Autodesk Inventor part; units mm, degrees
ref_plane "YZ Plane" through (0, 0, 0) normal (1, 0, 0) x (0, 1, 0)
ref_plane "XZ Plane" through (0, 0, 0) normal (0, 1, 0) x (-1, 0, 0)
ref_plane "XY Plane" through (0, 0, 0) normal (0, 0, 1) x (1, 0, 0)
sketch "Boceto1" plane through (-15.751, -17.109, 5) normal (0, 0, 1) x (1, 0, 0)
  line L0 (0, 0) -> (8.574, 5.146)
  circle A0 centre (4.287, 2.573) radius 4.9998
  point P0 (15.751, 17.109)
extrude "Extrusión1" add sketch "Boceto1" along normal blind 2
sketch "Boceto2" plane through (-11.464, -14.536, 7) normal (0, 0, 1) x (1, 0, 0)
  circle A0 centre (0, 0) radius 3.75
  point P0 (11.464, 14.536)
  dimension "d2" = 7.5
extrude "Extrusión2" add sketch "Boceto2" along normal blind 11
sketch "Boceto3" plane through (-11.464, -14.536, 18) normal (0, 0, 1) x (1, 0, 0)
  circle A0 centre (0, 0) radius 4.9998
  point P0 (11.464, 14.536)
extrude "Extrusión3" add sketch "Boceto3" along normal blind 2
sketch "Boceto4" plane through (-11.464, -14.536, 20) normal (0, 0, 1) x (1, 0, 0)
  circle A0 centre (0, 0) radius 2.5
  point P0 (11.464, 14.536)
  dimension "d7" = 5
extrude "Extrusión4" cut sketch "Boceto4" against normal blind 22
sketch "Boceto5" plane through (0, 0, 0) normal (1, 0, 0) x (0, 1, 0)
  line L0 (-18.286, 7) -> (-10.786, 7)
  line L1 (-14.536, 7) -> (-14.536, 8.5)
  line L2 (-14.536, 8.5) -> (-14.536, 18)
  line L3 (-10.786, 18) -> (-18.286, 18)
  line L4 (-14.536, 18) -> (-14.536, 16.5)
  circle A0 centre (-14.536, 16.5) radius 1
  circle A1 centre (-14.536, 8.5) radius 1
  point P0 (0, 0)
  dimension "d10" = 1.5
  dimension "d11" = 1.5
  dimension "d12" = 2
  dimension "d13" = 2
extrude "Extrusión5" cut sketch "Boceto5" against normal blind 22
sketch "Boceto7" plane through (-15.751, -17.109, 5) normal (0, 0, 1) x (1, 0, 0)
  circle A0 centre (4.287, 2.573) radius 2.5
  circle A1 centre (4.287, 2.573) radius 2.5
  point P0 (15.751, 17.109)
extrude "Extrusión6" add sketch "Boceto7" against normal blind 5
sketch "Boceto8" plane through (-11.464, -14.536, 0) normal (0, 0, -1) x (-1, 0, 0)
  circle A0 centre (0, 0) radius 2.5
  point P0 (-11.464, 14.536)
extrude "Extrusión7" cut sketch "Boceto8" against normal blind 5
properties part number "eng_chic_2_1"
For this review, take the finished solid that the model builds, in its own axes (mm). A direction names the side the tool comes from. Coordinates: 2 decimals unless noted, no trailing zeros. Write each loop counter-clockwise with the first axis right and the second up, starting at its lowest first coordinate (ties: lowest second). Pieces come first, ordered by that corner, then holes. Notation, with made-up numbers: (65.5, 0.5) -> (114.5, 0.5) arc R29 ccw to (114.5, 34.5) -> close; hole circle Ø6 at (-18.75, 47). An arc over 180 degrees is marked (long way). Put each result on its own line as item: value.
Q1. Take a section at B-B, the plane z = 17. State the section outline as (x, y) points.
From the geometry:
outline: (-15.11, -15.4) arc R3.75 ccw to (-7.82, -15.4) -> (-9.12, -15.4) arc R2.5 cw to (-13.81, -15.4) -> close; (-15.11, -13.67) -> (-13.81, -13.67) arc R2.5 cw to (-9.12, -13.67) -> (-7.82, -13.67) arc R3.75 ccw to start
Q2. Wall thickness on L1, parallel to Z at x = -8.75, y = -17.25; L2, parallel to Z at x = -15, y = -14.25; L3, parallel to X at y = -14.5, z = 17.75: over which ranges is each line inside the solid? List them lowest first.
From the geometry:
L1: z = 5 to 7, 18 to 20
L2: z = 5 to 7.54, 9.46 to 15.54, 17.46 to 20
L3: x = -15.21 to -13.96, -8.96 to -7.71
Q3. Take a section at D-D, the plane y = -15. Count the separate pieces of the cut face and the enclosed holes in it, then the cut area to 3 significant figures.
From the geometry:
separate pieces: 6
enclosed holes: 0
area: 39.0 mm2
Q4. Clearance check with flat-ended pins moving along their axes: pin 1 Ø2 at (x, z) = (-13, 18.5) entering from -Y; pin 2 Ø3 at (x, z) = (-12, 15) entering from +Y; pin 3 Ø3 at (y, z) = (-12.5, 13.5) entering from +X. State where each tip first meets the part, or that it passes through.
From the geometry:
pin 1: stops at y = -19.51
pin 2: stops at y = -10.79
pin 3: stops at x = -7.75
Q5. Take a section at A-A, the plane y = -10.5. State the section outline as (x, z) points.
From the geometry:
outline: (-14.42, 5) -> (-8.51, 5) -> (-8.51, 7) -> (-14.42, 7) -> close; (-14.42, 18) -> (-8.51, 18) -> (-8.51, 20) -> (-14.42, 20) -> close
Q6. Take a section at C-C, the plane x = -11.25. State the section outline as (y, z) points.
From the geometry:
outline: (-19.53, 5) -> (-17.03, 5) -> (-17.03, 20) -> (-19.53, 20) -> (-19.53, 18) -> (-18.28, 18) -> (-18.28, 7) -> (-19.53, 7) -> close; (-12.05, 5) -> (-9.54, 5) -> (-9.54, 7) -> (-10.79, 7) -> (-10.79, 18) -> (-9.54, 18) -> (-9.54, 20) -> (-12.05, 20) -> close
Q7. Tool access review of faces 4 (the cylindrical face through (-8, -13.1, 12.4)), 5 (the cylindrical face through (-8.4, -14.1, 15.6)): name each direction out of +Z, -Z, +X, -X, +Y, -Y from which nothing blocks a thin tool from reaching the whole face with its end or side.
From the geometry:
face 4: none
face 5: +X, -X
Q8. The part is to be moulded in two halves that separate along X. For faces 1 (the cylindrical face through (-14.474, -13.998, 9.343)), 2 (the cylindrical face through (-15, -11, 6)), 3 (the cylindrical face through (-9.155, -15.494, 12.605)), say which applies: +X half, -X half, draft (parallel to the pull), parting line (faces both ways), or undercut.
From the geometry:
face 1: draft
face 2: parting line
face 3: undercut
